The listing builds one solid part. Answer for the finished solid, in the listing's coordinates (mm). Face numbers are marked on the shaded views. A direction names the side the tool comes from. Round coordinates to 2 decimals unless told otherwise and drop trailing zeros. Order: outer loops, then holes, each group sorted by start corner. A loop starts at its lowest first (then second) coordinate and runs counter-clockwise, first axis right, second up. Notation, with made-up numbers: (-21.5, 7) - (21.5, 7) arc R34 ccw to (21.5, 43) - close; hole circle Ø11 at (74.25, 24). An arc over 180 degrees is marked (long way). Write item = value, one per line.
from build123d import *

# Parameters (mm, degrees)
SKETCH_2_W          = 25
SKETCH_2_H          = 25
EXTRUDE_1_DEPTH     = 3
SKETCH_3_R          = 1.5
CUT_EXTRUDE_2_DEPTH = 4
EXTRUDE_START       = -3
SKETCH_4_R          = 10
EXTRUDE_2_DEPTH     = 52
SKETCH_5_R          = 3.05
EXTRUDE_3_DEPTH     = 12


with BuildPart() as part:
    # 草图2 → 凸台-拉伸1 (new body)
    with BuildSketch(Plane.XY):
        with Locations((12.5, -12.5)):
            Rectangle(SKETCH_2_W, SKETCH_2_H)
    extrude(amount=EXTRUDE_1_DEPTH)

    # 草图3 → 切除-拉伸2 (cut, through all)
    with BuildSketch(Plane(origin=(0, 0, 0), x_dir=(-1, 0, 0), z_dir=(0, 0, -1))):
        with Locations((-22, -3)):
            Circle(SKETCH_3_R)
        with Locations((-3, -3)):
            Circle(SKETCH_3_R)
        with Locations((-3, -22)):
            Circle(SKETCH_3_R)
        with Locations((-22, -22)):
            Circle(SKETCH_3_R)
    extrude(amount=-CUT_EXTRUDE_2_DEPTH, mode=Mode.SUBTRACT)

    # 草图4 → 凸台-拉伸2 (add)
    with BuildSketch(Plane.XY.offset(3).offset(EXTRUDE_START)):
        with Locations((12.5, -12.5)):
            Circle(SKETCH_4_R)
    extrude(amount=-EXTRUDE_2_DEPTH)

    # 草图5 → 凸台-拉伸3 (add)
    with BuildSketch(Plane(origin=(0, 0, -52), x_dir=(-1, 0, 0), z_dir=(0, 0, -1))):
        with Locations((-12.5, -12.5)):
            Circle(SKETCH_5_R)
    extrude(amount=EXTRUDE_3_DEPTH)


solid = part.part
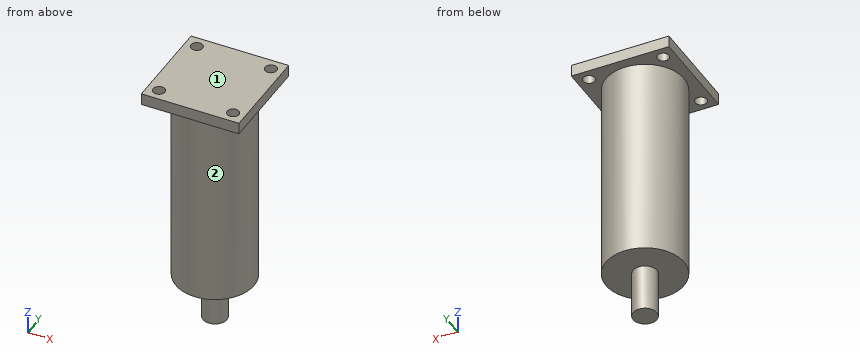
Q1. Flat-ended cylindrical pins translate along their axes: P1, Ø6, axis at x = 16, z = -40, coming from the -Y side; P2, Ø1.5, axis at x = 12, y = -5.5, coming from the -Z side; P3, Ø5, axis at x = 3, y = -3, coming from the -Z side; P4, Ø2.5, axis at x = 22, y = -3, coming from the -Z side. Find the tip coordinate at first contact, or state that the pin passes through.
Model answer:
P1 = -22.49
P2 = -52
P3 = 0
P4 = through
Q2. Find the intervals of material crossed by line 1 (Y direction, x = 22, z = 1); line 2 (Z direction, x = 2.25, y = -10.25); line 3 (Z direction, x = 14, y = -8.75), in increasing order. Write a range as from..to.
Model answer:
line_1 = -25..-23.5, -20.5..-4.5, -1.5..0
line_2 = 0..3
line_3 = -52..3
Q3. Section A-A on x = 12.5 is taken. Determine the outline of the cut face in (y, z).
Model answer:
outline = (-25, 0) - (-22.5, 0) - (-22.5, -52) - (-15.55, -52) - (-15.55, -64) - (-9.45, -64) - (-9.45, -52) - (-2.5, -52) - (-2.5, 0) - (0, 0) - (0, 3) - (-25, 3) - close
Q4. Section C-C on x = 21.25 is taken. Determine the outline of the cut face in (y, z), then the cut area to 3 significant figures.
Model answer:
outline = (-25, 0) - (-23.3, 0) - (-23.3, 3) - (-25, 3) - close; (-20.7, 0) - (-17.34, 0) - (-17.34, -52) - (-7.66, -52) - (-7.66, 0) - (-4.3, 0) - (-4.3, 3) - (-20.7, 3) - close; (-1.7, 0) - (0, 0) - (0, 3) - (-1.7, 3) - close
area = 563 mm^2
Q5. Section B-B on y = -12.5 is taken. Determine the outline of the cut face in (x, z), then the cut area to 3 significant figures.
Model answer:
outline = (0, 0) - (2.5, 0) - (2.5, -52) - (9.45, -52) - (9.45, -64) - (15.55, -64) - (15.55, -52) - (22.5, -52) - (22.5, 0) - (25, 0) - (25, 3) - (0, 3) - close
area = 1,190 mm^2
Q6. Section D-D on z = -13 is taken. Determine the outline of the cut face in (x, y), then the cut area to 3 significant figures.
Model answer:
outline = circle Ø20 at (12.5, -12.5)
area = 314 mm^2
Q7. For the marked faces 1 and 2, determine the directions among +Z, -Z, +X, -X, +Y, -Y from which every point of the face is accessible in a straight line to the end or side of a thin tool.
Model answer:
face_1 = +Z, +X, -X, +Y, -Y
face_2 = -Z
